Part model, mm, in its own coordinate system. Give positions to 0.01 mm unless a question says otherwise; leave off trailing zeros. Write each loop counter-clockwise with the first axis right and the second up, starting at its lowest first coordinate (ties: lowest second). Pieces come first, ordered by that corner, then holes.
```python
from build123d import *

# Parameters (mm, degrees)
F0_R          = 8.65
F1_DEPTH      = 2.25
F1_DEPTH_BACK = 2.25


# Not quite as in the source:
# - the program builds the solid bodies; features that only make, move or delete a surface that nothing else refers to are left out


with BuildPart() as f1:
    # F0 (on Front) → F1 (new body, two sides)
    with BuildSketch(Plane.XZ) as f1_sk:
        with BuildLine():
            ThreePointArc((-11.15, 0), (0, -11.15), (11.15, 0))
            ThreePointArc((11.15, 0), (7.8842406102, 7.8842406102), (0, 11.15))
            ThreePointArc((0, 11.15), (-7.8842406102, 7.8842406102), (-11.15, 0))
        make_face()
        Circle(F0_R, mode=Mode.SUBTRACT)
        with BuildLine():
            ThreePointArc((-11.15, 0), (-7.8842406102, 7.8842406102), (0, 11.15))
            Line((0, 11.15), (-4, 11.15))
            Line((-4, 11.15), (-9.15, 11.15))
            Line((-9.15, 11.15), (-11.15, 11.15))
            Line((-11.15, 11.15), (-11.15, 0))
        make_face()
        with BuildLine():
            ThreePointArc((0, 11.15), (7.8842406102, 7.8842406102), (11.15, 0))
            Line((11.15, 0), (11.15, 11.15))
            Line((11.15, 11.15), (0, 11.15))
        make_face()
    extrude(amount=F1_DEPTH)
    extrude(f1_sk.sketch, amount=-F1_DEPTH_BACK)


solid = f1.part
```
1) Saw through at D-D, the plane z = -9.25. Write the cut outline in (x, y), then the cut area to 3 significant figures.
Answers follow:
outline: (-6.23, -2.25) - (6.23, -2.25) - (6.23, 2.25) - (-6.23, 2.25) - close
area: 56.0 mm2
2) Saw through at B-B, the plane z = 0.5. Write the cut outline in (x, y).
Answers follow:
outline: (-11.15, -2.25) - (-8.64, -2.25) - (-8.64, 2.25) - (-11.15, 2.25) - close; (8.64, -2.25) - (11.15, -2.25) - (11.15, 2.25) - (8.64, 2.25) - close
3) Wall check: L1, parallel to Z at x = 0, y = 0.7; L2, parallel to X at y = 0.05, z = -7.75; L3, parallel to X at y = 1.85, z = 6.5. Give the ranges that are in metal, low to high.
Answers follow:
L1: z = -11.15 to -8.65, 8.65 to 11.15
L2: x = -8.02 to -3.84, 3.84 to 8.02
L3: x = -11.15 to -5.71, 5.71 to 11.15
4) Saw through at A-A, the plane x = 0. Write the cut outline in (y, z), then the cut area to 3 significant figures.
Answers follow:
outline: (-2.25, -11.15) - (2.25, -11.15) - (2.25, -8.65) - (-2.25, -8.65) - close; (-2.25, 8.65) - (2.25, 8.65) - (2.25, 11.15) - (-2.25, 11.15) - close
area: 22.5 mm2
5) Saw through at C-C, the plane y = 1.45. Write the cut outline in (x, z).
Answers follow:
outline: (-11.15, 0) arc R11.15 ccw to (11.15, 0) - (11.15, 11.15) - (-11.15, 11.15) - close; hole circle Ø17.3 at (0, 0)
6) Two-plate mould, pull along Z, no slides. Class faces 1 (the face through (8.25, 0.03, 2.6)), 2 (the face through (-0.245, -0.031, -11.147)), 3 (the face through (-11.15, 0, 6)): +Z half, -Z half, draft (parallel to the pull), parting line (faces both ways), or undercut.
Answers follow:
face 1: undercut
face 2: -Z half
face 3: draft
7) Pin check, flat tips, straight feed: pin 1 Ø10.5 at (x, z) = (0, 0) entering from +Y; pin 2 Ø10 at (x, z) = (8.5, 0.5) entering from -Y. Stop position of each tip, or through.
Answers follow:
pin 1: passes through
pin 2: stops at y = -2.25
